```python
from build123d import *

# Parameters (mm, degrees)
EXTRUDE_1_DEPTH     = 45
EXTRUDE_START       = -5
EXTRUDE_2_DEPTH     = 5
SKETCH_4_W          = 56.099400369
SKETCH_4_H          = 117.099049564
CUT_EXTRUDE_1_DEPTH = 68.024249343
SKETCH_8_R          = 1.6
CUT_EXTRUDE_3_DEPTH = 78.530639105
SKETCH_10_W         = 6
SKETCH_10_H         = 45
EXTRUDE_5_DEPTH     = 26
CUT_EXTRUDE_4_DEPTH = 31
EXTRUDE_6_DEPTH     = 45
CUT_EXTRUDE_6_DEPTH = 8
CUT_EXTRUDE_7_REACH = 82.1
SKETCH_19_R         = 1.5


with BuildPart() as part:
    # Sketch 1 → Extrude 1 (new body)
    with BuildSketch(Plane(origin=(0, 0, 0), x_dir=(1, 0, 0), z_dir=(0, 1, 0))):
        with BuildLine():
            Line((26, 55), (31, 55))
            ThreePointArc((31, 55), (26.606601718, 44.393398282), (16, 40))
            Line((16, 40), (10, 40))
            ThreePointArc((10, 40), (6.464466094, 38.535533906), (5, 35))
            Line((5, 35), (5, -35))
            ThreePointArc((5, -35), (6.464466094, -38.535533906), (10, -40))
            Line((10, -40), (16, -40))
            ThreePointArc((16, -40), (26.606601718, -44.393398282), (31, -55))
            Line((31, -55), (26, -55))
            ThreePointArc((26, -55), (23.071067812, -47.928932188), (16, -45))
            Line((16, -45), (10, -45))
            ThreePointArc((10, -45), (2.928932188, -42.071067812), (0, -35))
            Line((0, -35), (0, 35))
            ThreePointArc((0, 35), (2.928932188, 42.071067812), (10, 45))
            Line((10, 45), (16, 45))
            ThreePointArc((16, 45), (23.071067812, 47.928932188), (26, 55))
        make_face()
    extrude_1 = extrude(amount=EXTRUDE_1_DEPTH)

    # Sketch 3 → Extrude 2 (add)
    with BuildSketch(Plane(origin=(0, 45, 0), x_dir=(1, 0, 0), z_dir=(0, 1, 0)).offset(EXTRUDE_START)):
        with BuildLine():
            Line((5, 27.623228275), (26, 27.623228275))
            Line((26, 27.623228275), (26, 55))
            ThreePointArc((26, 55), (23.071067812, 47.928932188), (16, 45))
            Line((16, 45), (10, 45))
            ThreePointArc((10, 45), (2.928932188, 42.071067812), (0, 35))
            Line((0, 35), (0, 27.623228275))
            Line((0, 27.623228275), (5, 27.623228275))
        make_face()
        with BuildLine():
            Line((0, -27.623228275), (5, -27.623228275))
            Line((5, -27.623228275), (26, -27.623228275))
            Line((26, -27.623228275), (26, -55))
            ThreePointArc((26, -55), (23.071067812, -47.928932188), (16, -45))
            Line((16, -45), (10, -45))
            ThreePointArc((10, -45), (2.928932188, -42.071067812), (0, -35))
            Line((0, -35), (0, -27.623228275))
        make_face()
    extrude_2 = extrude(amount=EXTRUDE_2_DEPTH)

    # Sketch 4 → Cut-Extrude 1 (cut, through all)
    with BuildSketch(Plane(origin=(0, 22.5, 0), x_dir=(-1, 0, 0), z_dir=(0, -1, 0))):
        with Locations((-12.373979196, 0.253461146)):
            Rectangle(SKETCH_4_W, SKETCH_4_H)
    extrude(amount=CUT_EXTRUDE_1_DEPTH, mode=Mode.SUBTRACT)

    # Mirror 5: Extrude 1, Extrude 2 across plane
    add(extrude_1.mirror(Plane.ZX.offset(22.5)))
    add(extrude_2.mirror(Plane.ZX.offset(22.5)))

    # Sketch 8 → Cut-Extrude 3 (cut, through all)
    with BuildSketch(Plane(origin=(0, 0, 0), x_dir=(-1, 0, 0), z_dir=(0, -1, 0))):
        with Locations(Location((-15, 33, 0), (0, 0, 90))):
            Circle(SKETCH_8_R)
        with Locations(Location((-15, -33, 0), (0, 0, 90))):
            Circle(SKETCH_8_R)
    extrude(amount=-CUT_EXTRUDE_3_DEPTH, mode=Mode.SUBTRACT)

    # Sketch 10 → Extrude 5 (add)
    with BuildSketch(Plane.ZY):
        with Locations((0, 22.5)):
            Rectangle(SKETCH_10_W, SKETCH_10_H)
    extrude(amount=-EXTRUDE_5_DEPTH)

    # Sketch 2198 → Cut-Extrude 4 (cut)
    with BuildSketch(Plane(origin=(0, 38, 0), x_dir=(1, 0, 0), z_dir=(0, 1, 0))):
        Polygon((0, -18), (0, -35), (21.171611629, -26.013184045), (21.171611629, -9.013184045), align=None)
        Polygon((0, 32.448593019), (0, 18), (15.97488762, 11.219062513), (21.171611629, 23.461777064), align=None)
    extrude(amount=-CUT_EXTRUDE_4_DEPTH, mode=Mode.SUBTRACT)

    # Sketch 15 → Extrude 6 (add)
    with BuildSketch(Plane(origin=(0, 0, 0), x_dir=(-1, 0, 0), z_dir=(0, -1, 0))):
        Polygon((-18.373024886, 3), (-24.373024886, 3), (-30.49016031, 17.411067961), (-25.406185199, 19.569087362), align=None)
        Polygon((-31.8885242, -21.464124551), (-24.373024886, -3), (-18.373024886, -3), (-27.285999932, -23.417780194), align=None)
    extrude(amount=-EXTRUDE_6_DEPTH)

    # Sketch 16 → Cut-Extrude 6 (cut)
    with BuildSketch(Plane(origin=(0, 0, 0), x_dir=(-1, 0, 0), z_dir=(0, -1, 0))):
        Polygon((-24.373024886, -3), (-18.373024886, -3), (-21.889605043, -11.284543681), (-26.973580154, -9.12652428), align=None)
        Polygon((-18.373024886, 3), (-21.889605043, 11.284543681), (-26.973580154, 9.12652428), (-24.373024886, 3), align=None)
    cut_extrude_6 = extrude(amount=-CUT_EXTRUDE_6_DEPTH, mode=Mode.SUBTRACT)

    # Mirror 6: Cut-Extrude 6 across plane
    add(cut_extrude_6.mirror(Plane(origin=(0, 22.5, 0), x_dir=(0, 0, 1), z_dir=(0, -1, 0))), mode=Mode.SUBTRACT)

    # Sketch 19 → Cut-Extrude 7 (cut, up to next)
    with BuildSketch(Plane(origin=(19.572965618, 0, 8.308230983), x_dir=(0.39073112848926966, 0, -0.9205048534524422), z_dir=(0.9205048534524422, 0, 0.39073112848926966)), mode=Mode.PRIVATE) as cut_extrude_7_sk1:
        with Locations((23.440427308, 41)):
            Circle(SKETCH_19_R)
    cut_extrude_7_tool1 = extrude(cut_extrude_7_sk1.sketch, amount=-CUT_EXTRUDE_7_REACH, mode=Mode.PRIVATE) & part.part
    # Sketch 19 → Cut-Extrude 7 (cut, up to next)
    with BuildSketch(Plane(origin=(19.572965618, 0, 8.308230983), x_dir=(0.39073112848926966, 0, -0.9205048534524422), z_dir=(0.9205048534524422, 0, 0.39073112848926966)), mode=Mode.PRIVATE) as cut_extrude_7_sk2:
        with Locations((23.440427308, 4)):
            Circle(SKETCH_19_R)
    cut_extrude_7_tool2 = extrude(cut_extrude_7_sk2.sketch, amount=-CUT_EXTRUDE_7_REACH, mode=Mode.PRIVATE) & part.part
    cut_extrude_7_1 = cut_extrude_7_tool1.solids().sort_by_distance((28.73187, 41, -13.268796))[0]
    add(cut_extrude_7_1, mode=Mode.SUBTRACT)
    cut_extrude_7_2 = cut_extrude_7_tool2.solids().sort_by_distance((28.73187, 4, -13.268796))[0]
    add(cut_extrude_7_2, mode=Mode.SUBTRACT)
    cut_extrude_7 = cut_extrude_7_1 + cut_extrude_7_2  # Cut-Extrude 7 as one shape, for the pattern or mirror that repeats it

    # Mirror 7: Cut-Extrude 7 across plane
    add(cut_extrude_7.mirror(Plane.XY), mode=Mode.SUBTRACT)


solid = part.part
```
Can you work these out from the model? Positions are in its coordinate system, mm. A direction names the side the tool comes from. Give positions to 0.01 mm unless a question says otherwise; leave off trailing zeros. Order: outer loops, then holes, each group sorted by start corner. A loop starts at its lowest first (then second) coordinate and runs counter-clockwise, first axis right, second up. Notation, with made-up numbers: M 85.5,-38 L 101.5,-38 A21 cw 101.5,-31 Z; hole C 77,49 d11. An arc over 180 degrees is marked long. One line per item, written item: value.
1) Please list where these lines run through material, in increasing order: line 1 along Z through (x, y) = (23, 15.5); line 2 along Y through (x, z) = (8, -37); line 3 along X through (y, z) = (2.9, 33).
Answer sheet:
line 1: z = -47.86 to -41.73, -13.9 to 13.6, 41.73 to 47.86
line 2: y = 0 to 5, 40 to 45
line 3: x = 0 to 13.4, 16.6 to 26
2) On a 3-axis mill with a long thin cutter (end or side, diameter ignored), from which of +Z, -Z, +X, -X, +Y, -Y can I reach the whole of each face in a straight line? I mean faces 5 (the face through (15, 3, 27.623)), 6 (the face through (2.535, 22.717, 16.924)), 7 (the face through (6, 23, 38)). Say none if no direction works.
Answer sheet:
face 5: +X, +Y, -Y
face 6: none
face 7: +X
3) I want a section at D-D, the plane z = -37.5. List the corners of the cut face in (x, y) for me.
Answer sheet:
outline: M 0.32,0 L 26,0 L 26,5 L 5.67,5 L 5.67,40 L 26,40 L 26,45 L 0.32,45 Z
4) We'd pull the mould along X, two halves only. Please class faces 1 (the face through (26.49, 22.82, 44.28)), 2 (the face through (26.773, 4.451, 15.655)), 3 (the face through (5, 23, 15)), 4 (the face through (15, 42, -27.623)): released by +X, released by -X, zero draft, split by the parting line, or undercut.
Answer sheet:
face 1: released by +X
face 2: undercut
face 3: undercut
face 4: zero draft
5) For P1, Ø5.5, axis at y = 43, z = 33, coming from the +X side; P2, Ø3, axis at x = 6, y = 28.5, coming from the -Z side; P3, Ø6.5, axis at x = 13.5, y = 20.5, coming from the -Z side, each with a flat end and sliding along its axis, tell me the tip position at first contact or that it passes through.
Answer sheet:
P1: stops at x = 26
P2: stops at z = -44.68
P3: stops at z = -45.03
6) I want a section at B-B, the plane x = 15. Count the separate pieces of the cut face and the enclosed holes in it, plus the area to 3 significant figures.
Answer sheet:
separate pieces: 7
enclosed holes: 0
area: 904 mm^2
7) I want a section at A-A, the plane x = 7.5. List the corners of the cut face in (y, z) for me.
Answer sheet:
outline: M 0,-44.68 L 45,-44.68 L 45,-27.62 L 40,-27.62 L 40,-39.33 L 5,-39.33 L 5,-27.62 L 0,-27.62 Z; M 0,-3 L 45,-3 L 45,3 L 0,3 Z; M 0,27.62 L 5,27.62 L 5,39.33 L 40,39.33 L 40,27.62 L 45,27.62 L 45,44.68 L 0,44.68 Z
